Here's how the part is built. I have some questions about the finished solid (model axes, mm). A direction names the side the tool comes from. Give positions to 0.01 mm unless a question says otherwise; leave off trailing zeros. Loops run counter-clockwise (first coordinate to the right, second up) from the corner with the lowest first, then second, coordinate; pieces in that order, holes last. Notation, with made-up numbers: (-25.5, 10.5) - (-10.5, 10.5) arc R16 cw to (-10.5, 18.5) - close; hole circle Ø8 at (30.25, 61). An arc over 180 degrees is marked (long way). Return JSON: item names as keys, results as strings. Group by question number.
(1) For P1, Ø1, axis at x = 5, z = 9, coming from the -Y side; P2, Ø8, axis at x = 20.5, z = 12, coming from the +Y side, each with a flat end and sliding along its axis, tell me the tip position at first contact or that it passes through.
(2) If we mould it in two halves opening along Z, with no side actions, what happens to faces 1 (the flat face through (13, 207, 0)), 2 (the flat face through (22.8, 204, 13)), 3 (the flat face through (12.62, 415.9, 24))? For each: released by +Z, released by -Z, zero draft, split by the parting line, or undercut.
(3) If we section it at B-B (x = 6.25): Please give me the cut outline in (y, z), then the cut area to 3 significant figures.
(4) If we section it at C-C (y = 221): Please give me the cut outline in (x, z).
(5) On a 3-axis mill with a long thin cutter (end or side, diameter ignored), from which of +Z, -Z, +X, -X, +Y, -Y can I reach the whole of each face in a straight line? I mean faces 4 (the flat face through (12.98, 4.1, 24)), 5 (the flat face through (13, 207, 2.8)). Say none if no direction works.
(6) I need wall thicknesses on probe 1 along X at (y, z) = (23, 11.25); probe 2 along X at (y, z) = (231.5, 2.25). Which ranges of each line are inside material? Lowest first, please. Write a range as [from, to].
(7) If we section it at A-A (z = 11): Please give me the cut outline in (x, y).
```python
from build123d import *

# Parameters (mm, degrees)
BOSS_EXTRUDE1_DEPTH     = 420
SKETCH3_W               = 20
SKETCH3_H               = 20
CUT_EXTRUDE1_DEPTH      = 1040.5
CUT_EXTRUDE3_DEPTH      = 422.396725189
CUT_EXTRUDE3_DEPTH_BACK = 422.396725189
CUT_EXTRUDE4_DEPTH      = 422.396725189
CUT_EXTRUDE4_DEPTH_BACK = 422.396725189


with BuildPart() as part:
    # Sketch1 → Boss-Extrude1 (new body)
    with BuildSketch(Plane(origin=(0, 0, 0), x_dir=(1, 0, 0), z_dir=(0, 1, 0))):
        with BuildLine():
            Line((2.8, 0), (22.8, 0))
            ThreePointArc((22.8, 0), (24.779898987, -0.820101013), (25.6, -2.8))
            Line((25.6, -2.8), (25.6, -22.8))
            ThreePointArc((25.6, -22.8), (24.779898987, -24.779898987), (22.8, -25.6))
            Line((22.8, -25.6), (2.8, -25.6))
            ThreePointArc((2.8, -25.6), (0.820101013, -24.779898987), (0, -22.8))
            Line((0, -22.8), (0, -2.8))
            ThreePointArc((0, -2.8), (0.820101013, -0.820101013), (2.8, 0))
        make_face()
    extrude(amount=BOSS_EXTRUDE1_DEPTH)

    # Sketch3 → Cut-Extrude1 (cut)
    with BuildSketch(Plane(origin=(0, 0, 0), x_dir=(-1, 0, 0), z_dir=(0, -1, 0))):
        with Locations((-12.8, -12.8)):
            Rectangle(SKETCH3_W, SKETCH3_H)
    extrude(amount=-CUT_EXTRUDE1_DEPTH, mode=Mode.SUBTRACT)

    # Sketch5 → Cut-Extrude3 (cut, two sides: drawn at the far end of the back side and taken through both)
    with BuildSketch(Plane.XY.offset(22.8).offset(-CUT_EXTRUDE3_DEPTH_BACK)):
        Polygon((835.480673532, -263.146182429), (25.6, 0), (0, 8.317944224), (-809.880673532, 271.464126652), (-1336.173038389, -1348.297220411), (309.188308674, -1882.907529492), align=None)
    extrude(amount=CUT_EXTRUDE3_DEPTH + CUT_EXTRUDE3_DEPTH_BACK, mode=Mode.SUBTRACT)

    # Sketch4 → Cut-Extrude4 (cut, two sides: drawn at the far end of the back side and taken through both)
    with BuildSketch(Plane.XY.offset(22.8).offset(-CUT_EXTRUDE4_DEPTH_BACK)):
        Polygon((-809.880673532, 683.146182429), (0, 420), (25.6, 411.682055776), (835.480673532, 148.535873348), (1361.773038389, 1768.297220411), (-283.588308674, 2302.907529492), align=None)
    extrude(amount=CUT_EXTRUDE4_DEPTH + CUT_EXTRUDE4_DEPTH_BACK, mode=Mode.SUBTRACT)


solid = part.part
```
Values:
{
 "1": {"P1": "through", "P2": "y = 412.59"},
 "2": {"face 1": "released by -Z", "face 2": "undercut", "face 3": "zero draft"},
 "3": {"outline": "(6.29, 0) - (417.97, 0) - (417.97, 2.8) - (6.29, 2.8) - close; (6.29, 22.8) - (417.97, 22.8) - (417.97, 25.6) - (6.29, 25.6) - close", "area": "2,310 mm2"},
 "4": {"outline": "(0, 2.8) arc R2.8 ccw to (2.8, 0) - (22.8, 0) arc R2.8 ccw to (25.6, 2.8) - (25.6, 22.8) arc R2.8 ccw to (22.8, 25.6) - (2.8, 25.6) arc R2.8 ccw to (0, 22.8) - close; hole (2.8, 2.8) - (22.8, 2.8) - (22.8, 22.8) - (2.8, 22.8) - close"},
 "5": {"face 4": "+Z, -Z, -X, -Y", "face 5": "+Y, -Y"},
 "6": {"probe 1": "[0, 2.8], [22.8, 25.6]", "probe 2": "[0.05, 25.55]"},
 "7": {"outline": "(0, 8.32) - (2.8, 7.41) - (2.8, 419.09) - (0, 420) - close; (22.8, 0.91) - (25.6, 0) - (25.6, 411.68) - (22.8, 412.59) - close"}
}
